CAD build for the part. Positions are in the model's coordinates, mm. Face numbers are marked on the shaded views. A direction names the side the tool comes from. Give positions to 0.01 mm unless a question says otherwise; leave off trailing zeros. Loops run counter-clockwise (first coordinate to the right, second up) from the corner with the lowest first, then second, coordinate; pieces in that order, holes last. Notation, with made-up numbers: M 52,-34 L 92,-34 A31 ccw 92,-2 Z; hole C 89,12 d7. An arc over 180 degrees is marked long. One line per question, with ' | ' between items.
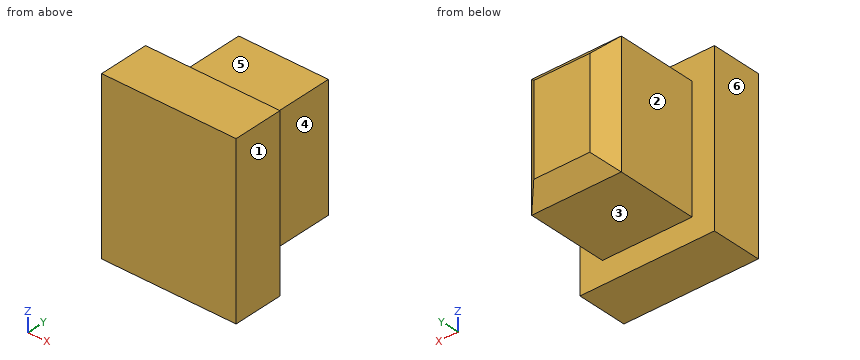
```python
from build123d import *

# Parameters (mm, degrees)
SKETCH_1_W      = 4.8
SKETCH_1_H      = 6
EXTRUDE_1_DEPTH = 1.8
SKETCH_2_W      = 3.2
SKETCH_2_H      = 4.4
EXTRUDE_2_DEPTH = 3.5
CHAMFER_1_SIZE  = 0.6


with BuildPart() as part:
    # 草图1 → 凸台-拉伸1 (new body)
    with BuildSketch(Plane(origin=(0, 0, 0), x_dir=(1, 0, 0), z_dir=(0, 1, 0))):
        with Locations((2.187378641, 1.04368932)):
            Rectangle(SKETCH_1_W, SKETCH_1_H)
    extrude(amount=EXTRUDE_1_DEPTH)

    # 草图2 → 凸台-拉伸2 (add)
    with BuildSketch(Plane(origin=(0, 1.8, 0), x_dir=(1, 0, 0), z_dir=(0, 1, 0))):
        with Locations((2.187378641, 1.04368932)):
            Rectangle(SKETCH_2_W, SKETCH_2_H)
    extrude(amount=EXTRUDE_2_DEPTH)

    # 倒角1
    chamfer_1_edges = [part.edges().sort_by_distance(p)[0] for p in [
        (2.187378641, 5.3, -3.24368932),
        (0.587378641, 5.3, -1.04368932),
        (2.187378641, 5.3, 1.15631068),
        (3.787378641, 5.3, -1.04368932),
    ]]
    chamfer(chamfer_1_edges, length=CHAMFER_1_SIZE)


solid = part.part
```
Item 1: Mould opens along X. For the marked faces 4, 5 and 6 say: pulls with the +X half, pulls with the -X half, needs draft (parallel to the pull), parting line crosses it, or undercut.
Conclusion:
face 4: pulls with the +X half | face 5: needs draft | face 6: pulls with the -X half
Item 2: 3-axis set-ups, long thin cutter, end or side, ignore diameter. For the marked faces 1, 2 and 3: which of +Z, -Z, +X, -X, +Y, -Y reach the whole face in a straight line?
Conclusion:
face 1: +Z, -Z, +X, +Y, -Y | face 2: +Z, -Z, -X, +Y | face 3: -Z, +X, -X, +Y
Item 3: Drop flat-ended pins along their axis: P1, Ø2.5, axis at x = 3, y = 4, coming from the -Z side; P2, Ø1.5, axis at x = 3, y = 3, coming from the +Z side; P3, Ø0.9, axis at y = 3, z = -1.5, coming from the -X side. Give the stop position or say it passes through.
Conclusion:
P1: z = -3.24 | P2: z = 1.16 | P3: x = 0.59
Item 4: Saw through at C-C on y = 3.65. Give the cut face in (x, z), and give its area (3 significant figures).
Conclusion:
outline: M 0.59,-3.24 L 3.79,-3.24 L 3.79,1.16 L 0.59,1.16 Z | area: 14.1 mm²
Item 5: Saw through at A-A on z = -2.4. Give the cut face in (x, y), and give its area (3 significant figures).
Conclusion:
outline: M -0.21,0 L 4.59,0 L 4.59,1.8 L 3.79,1.8 L 3.79,4.7 L 3.19,5.3 L 1.19,5.3 L 0.59,4.7 L 0.59,1.8 L -0.21,1.8 Z | area: 19.5 mm²
Item 6: Drill centre lines: line 1 along X through (y, z) = (4.5, -2.5); line 2 along Y through (x, z) = (3.65, 1.5); line 3 along Z through (x, y) = (3.55, 4.15). Where is each one in solid material? Low to high. Write a range as [from, to].
Conclusion:
line 1: [0.59, 3.79] | line 2: [0, 1.8] | line 3: [-3.24, 1.16]
Item 7: Saw through at B-B on x = 2.4. Give the cut face in (y, z), and give its area (3 significant figures).
Conclusion:
outline: M 0,-4.04 L 1.8,-4.04 L 1.8,-3.24 L 4.7,-3.24 L 5.3,-2.64 L 5.3,0.56 L 4.7,1.16 L 1.8,1.16 L 1.8,1.96 L 0,1.96 Z | area: 25.8 mm²
Item 8: Saw through at D-D on x = 0.1. Give the cut face in (y, z), and give its area (3 significant figures).
Conclusion:
outline: M 0,-4.04 L 1.8,-4.04 L 1.8,1.96 L 0,1.96 Z | area: 10.8 mm²
